Can you work these out from the model? Positions are in its coordinate system, mm. Give positions to 0.01 mm unless a question says otherwise; leave off trailing zeros. Loops run counter-clockwise (first coordinate to the right, second up) from the corner with the lowest first, then second, coordinate; pieces in that order, holes last. Notation, with made-up numbers: (75.5, -15.75) - (91.5, -15.75) arc R30 ccw to (91.5, 10.25) - close; hole circle Ø10 at (18, 68.25). An arc over 180 degrees is marked (long way). Answer as a JSON object with one key per item and string values.
```python
from build123d import *

# Parameters (mm, degrees)
SKETCH2_R           = 4.5
SKETCH2_R_2         = 2.5
SKETCH2_R_3         = 39
BOSS_EXTRUDE1_DEPTH = 5
BOSS_EXTRUDE2_START = -5
SKETCH3_R           = 39
SKETCH3_R_2         = 32.15
BOSS_EXTRUDE2_DEPTH = 5
SKETCH4_W           = 10
SKETCH4_H           = 120
CUT_EXTRUDE1_DEPTH  = 247.902363645
FILLET1_R           = 10


with BuildPart() as part:
    # Sketch2 → Boss-Extrude1 (new body)
    with BuildSketch(Plane.XY):
        Polygon((79.677872198, 233.639067486), (-60.322127802, 233.639067486), (-60.322127802, 223.639067486), (-60.322127802, 113.639067486), (79.677872198, 113.639067486), align=None)
        with Locations((-40.322127802, 123.639067486)):
            Circle(SKETCH2_R, mode=Mode.SUBTRACT)
        with Locations((-37.822127802, 156.139067486)):
            Circle(SKETCH2_R_2, mode=Mode.SUBTRACT)
        with Locations((59.677872198, 123.639067486)):
            Circle(SKETCH2_R, mode=Mode.SUBTRACT)
        with Locations((57.177872198, 156.139067486)):
            Circle(SKETCH2_R_2, mode=Mode.SUBTRACT)
        with Locations((-37.822127802, 191.139067486)):
            Circle(SKETCH2_R_2, mode=Mode.SUBTRACT)
        with Locations((9.677872198, 173.639067486)):
            Circle(SKETCH2_R_3, mode=Mode.SUBTRACT)
        with Locations((-40.322127802, 223.639067486)):
            Circle(SKETCH2_R, mode=Mode.SUBTRACT)
        with Locations((57.177872198, 191.139067486)):
            Circle(SKETCH2_R_2, mode=Mode.SUBTRACT)
        with Locations((59.677872198, 223.639067486)):
            Circle(SKETCH2_R, mode=Mode.SUBTRACT)
    extrude(amount=BOSS_EXTRUDE1_DEPTH)

    # Sketch3 → Boss-Extrude2 (add)
    with BuildSketch(Plane.XY.offset(5).offset(BOSS_EXTRUDE2_START)):
        with Locations((9.677872198, 173.639067486)):
            Circle(SKETCH3_R)
        with Locations((9.677872198, 173.639067486)):
            Circle(SKETCH3_R_2, mode=Mode.SUBTRACT)
    extrude(amount=BOSS_EXTRUDE2_DEPTH)

    # Sketch4 → Cut-Extrude1 (cut, through all)
    with BuildSketch(Plane.XY.offset(5)):
        with Locations((74.677872198, 173.639067486)):
            Rectangle(SKETCH4_W, SKETCH4_H)
        with Locations((-55.322127802, 173.639067486)):
            Rectangle(SKETCH4_W, SKETCH4_H)
    extrude(amount=-CUT_EXTRUDE1_DEPTH, mode=Mode.SUBTRACT)

    # Fillet1
    fillet1_edges = [part.edges().sort_by_distance(p)[0] for p in [
        (-50.322127802, 233.639067486, 2.5),
        (-50.322127802, 113.639067486, 2.5),
        (69.677872198, 113.639067486, 2.5),
        (69.677872198, 233.639067486, 2.5),
    ]]
    fillet(fillet1_edges, radius=FILLET1_R)


solid = part.part
```
1) I need wall thicknesses on L1, parallel to Y at x = -42, z = 3.3; L2, parallel to X at y = 175, z = 4.65; L3, parallel to X at y = 227.5, z = 1.45. Which ranges of each line are inside material? Lowest first, please.
Check sheet entries:
{"L1": "113.78 to 119.46, 127.81 to 219.46, 227.81 to 233.5", "L2": "-50.32 to -22.44, 41.8 to 69.68", "L3": "-49.55 to -42.63, -38.01 to 57.37, 61.99 to 68.9"}
2) Imagine slicing it at B-B on y = 161.5. Write out the boundary of the cut face in (x, z).
Check sheet entries:
{"outline": "(-50.32, 0) - (-20.09, 0) - (-20.09, 5) - (-50.32, 5) - close; (39.45, 0) - (69.68, 0) - (69.68, 5) - (39.45, 5) - close"}
3) If we mould it in two halves opening along Y, with no side actions, what happens to faces 1 (the cylindrical face through (24.513, 145.116, 2.465)), 2 (the cylindrical face through (66.83, 116.65, 2.46)), 3 (the cylindrical face through (59.1, 228.1, 2.5)), 4 (the flat face through (69.678, 173, 3))? For each: released by +Y, released by -Y, zero draft, split by the parting line, or undercut.
Check sheet entries:
{"face 1": "undercut", "face 2": "released by -Y", "face 3": "undercut", "face 4": "zero draft"}
4) I'm going to push a flat-ended pin straight in: P1, Ø8, axis at x = -40.32, y = 223.64, coming from the +Z side. Where does the tip first touch, or does it pass through?
Check sheet entries:
{"P1": "through"}
5) Imagine slicing it at A-A on x = -5.5. Write out the boundary of the cut face in (y, z).
Check sheet entries:
{"outline": "(113.64, 0) - (145.3, 0) - (145.3, 5) - (113.64, 5) - close; (201.98, 0) - (233.64, 0) - (233.64, 5) - (201.98, 5) - close"}
6) Imagine slicing it at C-C on z = 2.3. Give the number of separate pieces and of enclosed holes in the cut face, and give its area (3 significant figures).
Check sheet entries:
{"separate pieces": "1", "enclosed holes": "9", "area": "10,700 mm2"}
